Drawing for the job (mm, zero at the part's lowest x, y, z). Round coordinates to 2 decimals unless told otherwise and drop trailing zeros. Write each loop counter-clockwise with the first axis right and the second up, starting at its lowest first coordinate (ties: lowest second). Pieces come first, ordered by that corner, then holes. Notation, with made-up numbers: (3.25, 55) -> (22.25, 55) arc R33 ccw to (22.25, 87) -> close; hole circle Ø2 at (3.25, 8). An arc over 180 degrees is marked (long way). One line per question, with ' | ' between items.
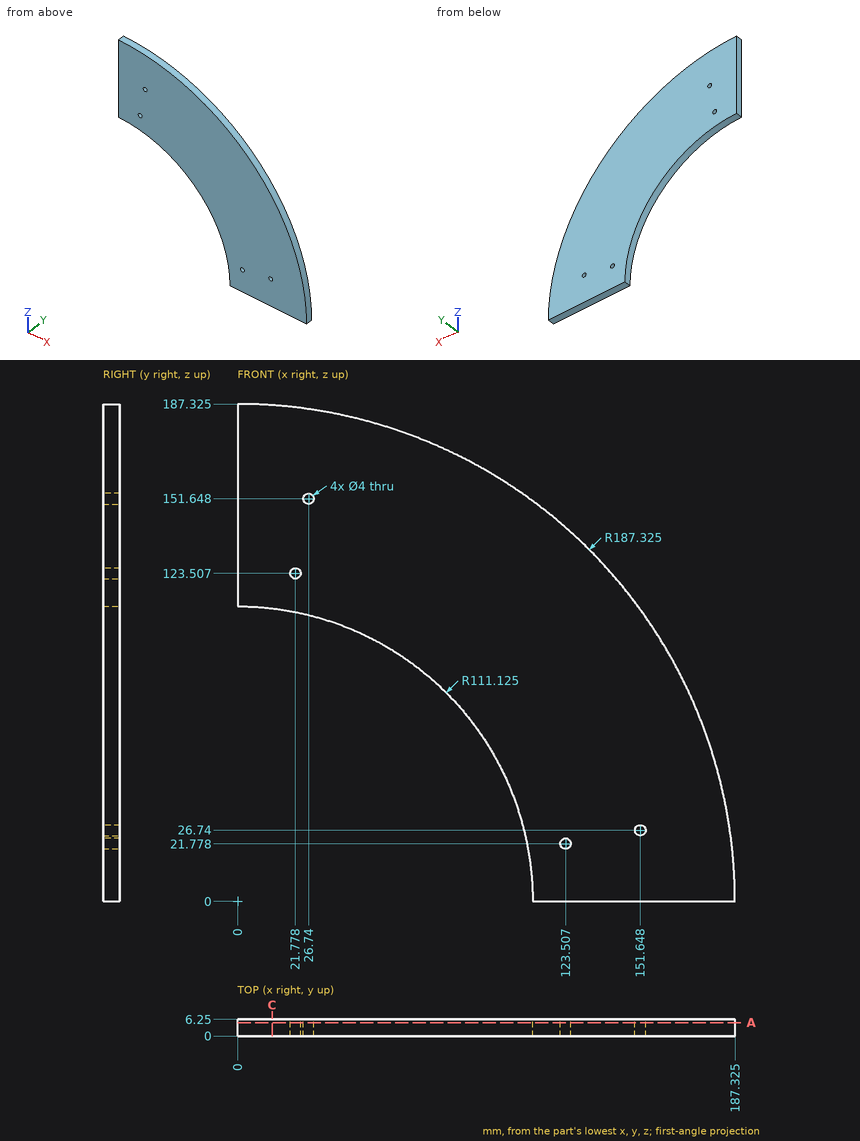
(1) Slice it at C-C (x = 13). Write the cut outline in (y, z).
Calculated:
outline: (0, 110.36) -> (6.25, 110.36) -> (6.25, 186.87) -> (0, 186.87) -> close
(2) Slice it at A-A (y = 5). State how many separate pieces and enclosed holes the cut face has, then the cut area to 3 significant figures.
Calculated:
separate pieces: 1 | enclosed holes: 4 | area: 17,800 mm2
(3) Drop flat-ended pins along their axis: pin 1 (1.5 mm diameter, centred on y = 4, z = 95, fed in from -X); pin 2 (3 mm diameter, centred on x = 21.78, z = 123.51, fed in from +Y); pin 3 (1.5 mm diameter, centred on y = 3.5, z = 128, fed in from +X); pin 4 (3 mm diameter, centred on y = 5, z = 158, fed in from +X). Give the stop position or say it passes through.
Calculated:
pin 1: x = 56.4 | pin 2: through | pin 3: x = 137.47 | pin 4: x = 102.95
(4) Wall check: line 1 (Z direction, x = 125, y = 4) (1 decimal); line 2 (Z direction, x = 20, y = 0.5) (1 decimal); line 3 (X direction, y = 1.25, z = 57.5). Give the ranges that are in metal, low to high. Write a range as from..to.
Calculated:
line 1: 0..20.4, 23.1..139.5 | line 2: 109.3..122.6, 124.4..186.3 | line 3: 95.09..178.28
